from build123d import *

# Parameters (mm, degrees)
F0_R     = 14.2875
F0_R_2   = 5.55625
F1_DEPTH = 12.7


with BuildPart() as f1:
    # F0 (on Top) → F1 (new body)
    with BuildSketch(Plane.XY):
        with BuildLine():
            ThreePointArc((25.4, -19.05), (30.120695, -10.040232), (31.75, 0))
            ThreePointArc((31.75, 0), (30.120695, 10.040232), (25.4, 19.05))
            ThreePointArc((25.4, 19.05), (0, 31.75), (-25.4, 19.05))
            ThreePointArc((-25.4, 19.05), (-31.75, 0), (-25.4, -19.05))
            ThreePointArc((-25.4, -19.05), (0, -31.75), (25.4, -19.05))
        make_face()
        Circle(F0_R, mode=Mode.SUBTRACT)
        with BuildLine():
            ThreePointArc((-25.4, -19.05), (-31.75, 0), (-25.4, 19.05))
            Line((-25.4, 19.05), (-57.94375, 9.525))
            ThreePointArc((-57.94375, 9.525), (-67.46875, 0), (-57.94375, -9.525))
            Line((-57.94375, -9.525), (-25.4, -19.05))
        make_face()
        with Locations((-57.94375, 0)):
            Circle(F0_R_2, mode=Mode.SUBTRACT)
        with BuildLine():
            ThreePointArc((25.4, 19.05), (30.120695, 10.040232), (31.75, 0))
            ThreePointArc((31.75, 0), (30.120695, -10.040232), (25.4, -19.05))
            Line((25.4, -19.05), (57.94375, -9.525))
            ThreePointArc((57.94375, -9.525), (67.46875, 0), (57.94375, 9.525))
            Line((57.94375, 9.525), (25.4, 19.05))
        make_face()
        with Locations((57.94375, 0)):
            Circle(F0_R_2, mode=Mode.SUBTRACT)
    extrude(amount=F1_DEPTH)


solid = f1.part
The listing builds one solid part. Answer for the finished solid, in the listing's coordinates (mm). Coordinates: 2 decimals unless noted, no trailing zeros. Write each loop counter-clockwise with the first axis right and the second up, starting at its lowest first coordinate (ties: lowest second). Pieces come first, ordered by that corner, then holes. Notation, with made-up numbers: (-19, -21.75) - (6, -21.75) arc R5 ccw to (6, -14.75) - close; hole circle Ø4 at (-35, 24). An arc over 180 degrees is marked (long way). Return JSON: item names as keys, results as strings.
1. The part is cut by section D-D on y = 8. Determine the outline of the cut face in (x, z).
Final values:
{"outline": "(-63.11, 0) - (-11.84, 0) - (-11.84, 12.7) - (-63.11, 12.7) - close; (11.84, 0) - (63.11, 0) - (63.11, 12.7) - (11.84, 12.7) - close"}
2. For a pull along X with two mould halves and no side action, classify faces 1 (the face through (-14.274, 0.628, 6.261)), 2 (the face through (41.444, -14.354, 6.261)), 3 (the face through (0.412, 31.747, 6.261)), 4 (the face through (-41.9, -14.22, 6.26)) as +X half, -X half, draft (parallel to the pull), parting line (faces both ways), or undercut.
Final values:
{"face 1": "undercut", "face 2": "+X half", "face 3": "parting line", "face 4": "-X half"}
3. The part is cut by section C-C on x = -9. Determine the outline of the cut face in (y, z), then the cut area to 3 significant figures.
Final values:
{"outline": "(-30.45, 0) - (-11.1, 0) - (-11.1, 12.7) - (-30.45, 12.7) - close; (11.1, 0) - (30.45, 0) - (30.45, 12.7) - (11.1, 12.7) - close", "area": "492 mm^2"}
4. The part is cut by section B-B on z = 4.25. Count the separate pieces of the cut face and the enclosed holes in it, then the cut area to 3 significant figures.
Final values:
{"separate pieces": "1", "enclosed holes": "3", "area": "4,150 mm^2"}
5. The part is cut by section A-A on y = 0. Determine the outline of the cut face in (x, z).
Final values:
{"outline": "(-67.47, 0) - (-63.5, 0) - (-63.5, 12.7) - (-67.47, 12.7) - close; (-52.39, 0) - (-14.29, 0) - (-14.29, 12.7) - (-52.39, 12.7) - close; (14.29, 0) - (52.39, 0) - (52.39, 12.7) - (14.29, 12.7) - close; (63.5, 0) - (67.47, 0) - (67.47, 12.7) - (63.5, 12.7) - close"}
6. Each of these flat-tipped pins is pushed along its axis until it touches: pin 1 Ø3 at (x, z) = (22.5, 10.5) entering from +Y; pin 2 Ø2 at (x, z) = (-4.5, 2.5) entering from -Y. Where does it stop, or does it pass through?
Final values:
{"pin 1": "y = 23.81", "pin 2": "y = -31.56"}
7. Consider line 1 along X through (y, z) = (5, 11.75); line 2 along X through (y, z) = (-4.5, 7.5); line 3 along Y through (x, z) = (-7, 1). Determine where each line is inside the solid, lowest interval first.
Final values:
{"line 1": "-66.05 to -60.37, -55.52 to -13.38, 13.38 to 55.52, 60.37 to 66.05", "line 2": "-66.34 to -61.2, -54.68 to -13.56, 13.56 to 54.68, 61.2 to 66.34", "line 3": "-30.97 to -12.46, 12.46 to 30.97"}
